Here's the drawing with two shaded views (mm, measured from the low corner). I have some questions. A direction names the side the tool comes from. Give positions to 0.01 mm unless a question says otherwise; leave off trailing zeros. Loops run counter-clockwise (first coordinate to the right, second up) from the corner with the lowest first, then second, coordinate; pieces in that order, holes last. Notation, with made-up numbers: M 36.5,65.25 L 40.5,65.25 A21 cw 40.5,72.25 Z; hole C 36,89 d2. An arc over 180 degrees is marked long. Answer in a Markdown table with one row per item. Add a question column.
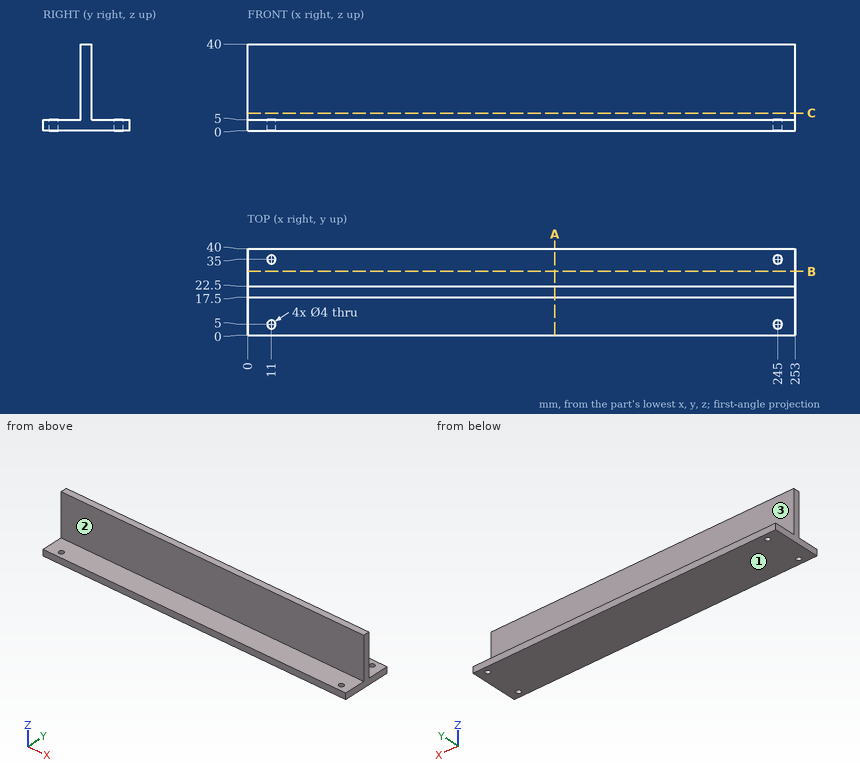
Item 1: Suppose I cut it at B-B (y = 29.5). List the corners of the cut face in (x, z) for me, then the cut area to 4 significant figures.
Item 2: Suppose I cut it at C-C (z = 8). List the corners of the cut face in (x, y) for me.
Item 3: For P1, Ø12, axis at x = 106.5, z = 9.5, coming from the -Y side; P2, Ø3.5, axis at x = 11, y = 35, coming from the +Z side; P3, Ø4, axis at x = 178.5, z = 23.5, coming from the -Y side; P4, Ø14, axis at x = 130.5, y = 6, coming from the +Z side, each with a flat end and sliding along its axis, tell me the tip position at first contact or that it passes through.
Item 4: Suppose I cut it at A-A (x = 142). List the corners of the cut face in (y, z) for me, then the cut area to 3 significant figures.
Item 5: For the marked faces 1, 2 and 3, which set-ups out of +Z, -Z, +X, -X, +Y, -Y let a thin tool reach every point of the face, with its end or its side?
Item 6: I need wall thicknesses on L1, parallel to X at y = 35, z = 1.6; L2, parallel to Y at x = 245, z = 3.35; L3, parallel to Y at x = 50.5, z = 21. Which ranges of each line are inside material? Lowest first, please.
Values found:
| question | item | result |
|---|---|---|
| 1 | outline | M 0,0 L 253,0 L 253,5 L 0,5 Z |
| 1 | area | 1,265 mm² |
| 2 | outline | M 0,17.5 L 253,17.5 L 253,22.5 L 0,22.5 Z |
| 3 | P1 | y = 0 |
| 3 | P2 | through |
| 3 | P3 | y = 17.5 |
| 3 | P4 | z = 5 |
| 4 | outline | M 0,0 L 40,0 L 40,5 L 22.5,5 L 22.5,40 L 17.5,40 L 17.5,5 L 0,5 Z |
| 4 | area | 375 mm² |
| 5 | face 1 | -Z, +X, -X, +Y, -Y |
| 5 | face 2 | +Z, +X, -X, -Y |
| 5 | face 3 | +Z, +X, -X, +Y |
| 6 | L1 | 0 to 9, 13 to 243, 247 to 253 |
| 6 | L2 | 0 to 3, 7 to 33, 37 to 40 |
| 6 | L3 | 17.5 to 22.5 |
